Check sheet for the modelled part. Datum: model origin and axes. Units: mm. Give positions to 0.01 mm unless a question says otherwise; leave off trailing zeros. Order: outer loops, then holes, each group sorted by start corner. A loop starts at its lowest first (then second) coordinate and runs counter-clockwise, first axis right, second up.
Item 1: Sectioned sample at B-B on x = 0. Record the boundary of the cut face in (y, z).
Item 2: Sectioned sample at C-C on y = 0.2. Record the boundary of the cut face in (x, z), and give its area (3 significant figures).
Item 3: Sectioned sample at D-D on z = 9.85. Record the boundary of the cut face in (x, y), and give its area (3 significant figures).
Item 4: Gauge pin test, flat ends, axial feed: P1, Ø0.5, axis at y = 0.5, z = 7.5, coming from the -X side; P2, Ø2, axis at x = -2, z = 4.5, coming from the -Y side. Record the tip position at first contact, or that the pin passes through.
Item 5: Material ranges on line 1 along Z through (x, y) = (0, 0.8); line 2 along X through (y, z) = (0.6, 9.85); line 3 along X through (y, z) = (0.7, 0), recorded low to high.
Item 6: Sectioned sample at A-A on z = 0. Record the boundary of the cut face in (x, y), and give its area (3 significant figures).
Autodesk Inventor part; units mm, degrees
ref_plane "YZ Plane" through (0, 0, 0) normal (1, 0, 0) x (0, 1, 0)
ref_plane "XZ Plane" through (0, 0, 0) normal (0, 1, 0) x (-1, 0, 0)
ref_plane "XY Plane" through (0, 0, 0) normal (0, 0, 1) x (1, 0, 0)
sketch "Sketch1" plane through (0, 0, 0) normal (0, 1, 0) x (-1, 0, 0)
  circle A0 centre (0, 0) radius 5.2
  line L0 (2, 12.5) -> (-2, 12.5)
  line L1 (-2, 12.5) -> (-2, -12.5)
  line L2 (-2, -12.5) -> (2, -12.5)
  line L3 (2, -12.5) -> (2, 12.5)
  line L4 (2, 12.5) -> (-2, -12.5) construction
  line L5 (-2, 12.5) -> (2, -12.5) construction
  line L6 (0, 12.5) -> (0, 9.85)
  line L7 (0, -12.5) -> (0, -9.85)
  point P0 (-2, 4.8)
  point P1 (-2, -4.8)
  point P2 (2, -4.8)
  point P3 (2, 4.8)
  dimension "d0" = 10.4
  dimension "d1" = 4
  dimension "d2" = 25
  dimension "d19" = 2.65
  dimension "d20" = 2.65
extrude "Extrusion1" add sketch "Sketch1" along normal blind 1
hole "Hole2" at (0, 0, 0) direction (0, 1, 0) diameter 7.4 depth 1 tip angle 118 countersink diameter 8.4 countersink angle 90
hole "Hole3" at (0, 0, 9.85) direction (0, 1, 0) diameter 2 depth 1 tip angle 118
hole "Hole4" at (0, 0, -9.85) direction (0, 1, 0) diameter 2 depth 1 tip angle 118
properties part number "Headplate_2p"
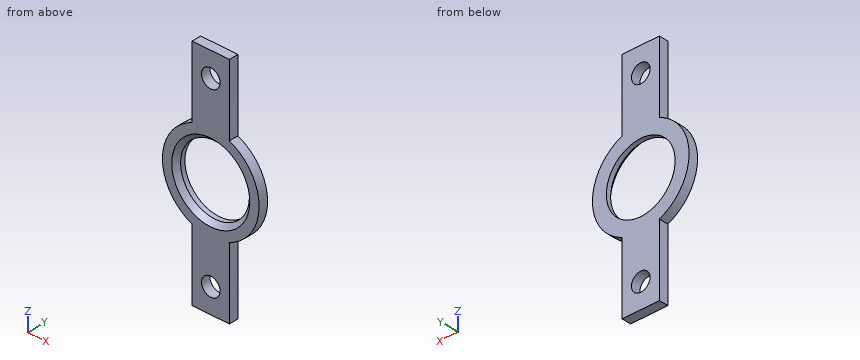
Report:
1. outline: (0, -12.5) - (1, -12.5) - (1, -10.85) - (0, -10.85) - close; (0, -8.85) - (1, -8.85) - (1, -3.7) - (0.5, -3.7) - (0, -4.2) - close; (0, 4.2) - (0.5, 3.7) - (1, 3.7) - (1, 8.85) - (0, 8.85) - close; (0, 10.85) - (1, 10.85) - (1, 12.5) - (0, 12.5) - close
2. outline: (-2, -12.5) - (2, -12.5) - (2, -4.8) arc R5.2 ccw to (2, 4.8) - (2, 12.5) - (-2, 12.5) - (-2, 4.8) arc R5.2 ccw to (-2, -4.8) - close; hole circle Ø8 at (0, 0); hole circle Ø2 at (0, -9.85); hole circle Ø2 at (0, 9.85)
2. area: 87.8 mm2
3. outline: (-2, 0) - (-1, 0) - (-1, 1) - (-2, 1) - close; (1, 0) - (2, 0) - (2, 1) - (1, 1) - close
3. area: 2.00 mm2
4. P1: stops at x = -2
4. P2: stops at y = 0
5. line 1: z = -12.5 to -10.85, -8.85 to -3.7, 3.7 to 8.85, 10.85 to 12.5
5. line 2: x = -2 to -1, 1 to 2
5. line 3: x = -5.2 to -3.7, 3.7 to 5.2
6. outline: (-5.2, 0) - (-4.2, 0) - (-3.7, 0.5) - (-3.7, 1) - (-5.2, 1) - close; (3.7, 0.5) - (4.2, 0) - (5.2, 0) - (5.2, 1) - (3.7, 1) - close
6. area: 2.75 mm2
